from build123d import *

# Parameters (mm, degrees)
F0_R     = 8.60044
F0_R_2   = 3.2004
F2_ANGLE = 90
F3_DEPTH = 25.4
F4_SIZE2 = 3.582964248
F4_SIZE  = 20.32
F5_W     = 290.7801419497
F5_H     = 55.9114702046
F6_DEPTH = 25.4


with BuildPart() as f2:
    # F0 (on Top) → F2 (revolve)
    with BuildSketch(Plane.XY):
        Circle(F0_R)
        Circle(F0_R_2, mode=Mode.SUBTRACT)
    revolve(axis=Axis((-12.7, -0.6994176656, 0), (0, -1, 0)), revolution_arc=F2_ANGLE)

    # F3 (add): a face of the model
    f3_faces = [f2.faces().sort_by_distance(p)[0] for p in [
        (-12.7, 0, 4.3428171778),
    ]]
    extrude(f3_faces, amount=F3_DEPTH)

    # F4
    f4_edges = [f2.edges().sort_by_distance(p)[0] for p in [
        (-38.1, 0, 9.4996),
    ]]
    f4_side = f2.faces().sort_by_distance((-25.4, 0, 9.4996))[0]
    chamfer(f4_edges, length=F4_SIZE, length2=F4_SIZE2, reference=f4_side)

    # F5 (on Front) → F6 (cut)
    with BuildSketch(Plane.XZ):
        with Locations((-2.42703408, 7.5079593807)):
            Rectangle(F5_W, F5_H)
    extrude(amount=-F6_DEPTH, mode=Mode.SUBTRACT)


solid = f2.part
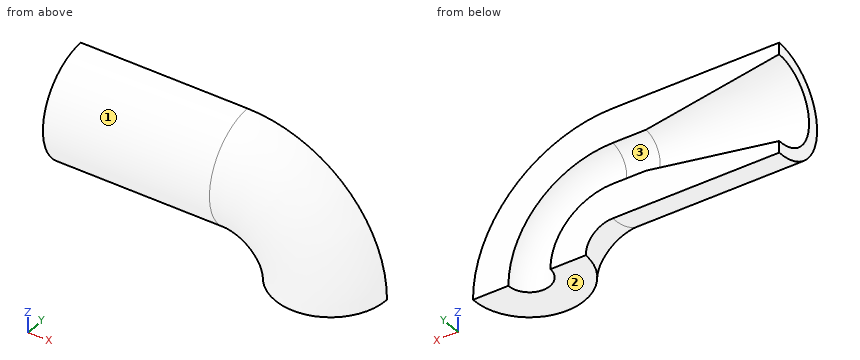
Can you work these out from the model? Positions are in its coordinate system, mm. Face numbers are marked on the shaded views. A direction names the side the tool comes from. Give positions to 0.01 mm unless a question says otherwise; leave off trailing zeros. Loops run counter-clockwise (first coordinate to the right, second up) from the corner with the lowest first, then second, coordinate; pieces in that order, holes last. Notation, with made-up numbers: M 30,69.5 L 68,69.5 A14 cw 68,94.5 Z; hole C -3,2.25 d6. An arc over 180 degrees is marked long. One line per item, written item: value. Start each with the question number.
1) If we section it at A-A, the plane y = -7.25: Write out the boundary of the cut face in (x, z), and give its area (3 significant figures).
2) If we section it at B-B, the plane x = -15: Write out the boundary of the cut face in (y, z), and give its area (3 significant figures).
3) I'm going to push flat-ended pins straight in: pin 1 (1 mm diameter, centred on x = -26.5, y = -7, fed in from -Z); pin 2 (6 mm diameter, centred on x = -26.5, z = 13, fed in from +Y); pin 3 (2 mm diameter, centred on x = -6.5, y = -2, fed in from +Z). Where does each tip first touch, or does it pass through?
4) If I drill on line 1 (Z direction, x = -18.5, y = -1); line 2 (Z direction, x = -24, y = -3.25); line 3 (Z direction, x = 5.5, y = -1), over which ranges is the centre line in solid material (lowest first)? Write a range as [from, to].
5) On a 3-axis mill with a long thin cutter (end or side, diameter ignored), from which of +Z, -Z, +X, -X, +Y, -Y can I reach the whole of each face in a straight line? I mean the marked faces 1, 2 and 3. Say none if no direction works.
Completed:
1. outline: M -38.1,8.07 L -12.7,8.07 A8.07 cw -4.63,0 L 4.63,0 A17.33 ccw -12.7,17.33 L -38.1,17.33 Z
1. area: 420 mm^2
2. outline: M 0,4.1 L 0,9.5 A3.2 cw 0,15.9 L 0,21.3 A8.6 ccw Z
2. area: 100 mm^2
3. pin 1: stops at z = 7.07
3. pin 2: stops at y = -3.31
3. pin 3: stops at z = 20.49
4. line 1: z = [4.16, 9.53], [15.87, 21.24]
4. line 2: z = [4.74, 9.89], [15.51, 20.66]
4. line 3: z = [0, 10.95]
5. face 1: -X, -Y
5. face 2: -Z, +X, -X, +Y, -Y
5. face 3: -X, +Y
